Here's how the part is built. I have some questions about the finished solid (model axes, mm). A direction names the side the tool comes from. Coordinates: 2 decimals unless noted, no trailing zeros. Write each loop counter-clockwise with the first axis right and the second up, starting at its lowest first coordinate (ties: lowest second). Pieces come first, ordered by that corner, then holes.
Item 1: I want a section at A-A (y = 1.5). Please give me the cut outline in (x, z), and give its area (3 significant figures).
Item 2: For faces 4 (the face through (-28.503, 11.843, 0.986)), 5 (the face through (2, 14, 0)), which set-ups out of +Z, -Z, +X, -X, +Y, -Y let a thin tool reach every point of the face, with its end or its side?
Item 3: I want a section at B-B (z = 0.8). Please give me the cut outline in (x, y) (3 decimals).
Item 4: I'm going to push flat-ended pins straight in: P1, Ø1, axis at x = -28.5, z = 0.5, coming from the +Y side; P2, Ø1, axis at x = -10, z = 0.5, coming from the -Y side; P3, Ø1, axis at x = -34.5, z = 1.5, coming from the +Y side. Where does each tip first touch, or does it pass through?
Item 5: If we mould it in two halves opening along X, with no side actions, what happens to faces 1 (the face through (2, 11.896, 1)), 2 (the face through (63.977, 4, 1)), 3 (the face through (2, 14, 2))? For each: pulls with the +X half, pulls with the -X half, needs draft (parallel to the pull), parting line crosses it, or undercut.
Item 6: I want a section at C-C (y = 7). Please give me the cut outline in (x, z).
Item 7: I want a section at D-D (x = -3). Please give me the cut outline in (y, z), and give its area (3 significant figures).
Item 8: Please list where these lines run through material, in increasing order: line 1 (X direction, y = 3.25, z = 1.45); line 2 (Y direction, x = 13, z = 0.8); line 3 (Y direction, x = 34.5, z = 0.9).
from build123d import *

# Parameters (mm, degrees)
SALIENTE_EXTRUIR1_DEPTH = 2


with BuildPart() as part:
    # Croquis1 → Saliente-Extruir1 (new body)
    with BuildSketch(Plane.XY):
        with BuildLine():
            Line((-27.468702439, 15.986263571), (30.422317404, 15.986263571))
            ThreePointArc((30.422317404, 15.986263571), (31.470993229, 15.931125511), (32.508104664, 15.766319374))
            Line((32.508104664, 15.766319374), (63.185386208, 9.223791978))
            ThreePointArc((63.185386208, 9.223791978), (63.754167993, 8.874841751), (63.976807482, 8.245786398))
            Line((63.976807482, 8.245786398), (63.976807482, 0.055005987))
            ThreePointArc((63.976807482, 0.055005987), (63.683914264, -0.652100794), (62.976807482, -0.944994013))
            Line((62.976807482, -0.944994013), (62.176807482, -0.944994013))
            ThreePointArc((62.176807482, -0.944994013), (61.469700701, -0.652100794), (61.176807482, 0.055005987))
            Line((61.176807482, 0.055005987), (61.176807482, 4.752984684))
            ThreePointArc((61.176807482, 4.752984684), (60.954167993, 5.382040037), (60.385386208, 5.730990264))
            Line((60.385386208, 5.730990264), (32.508104664, 11.67636316))
            ThreePointArc((32.508104664, 11.67636316), (31.470993229, 11.841169298), (30.422317404, 11.896307357))
            Line((30.422317404, 11.896307357), (-27.468702439, 11.896307357))
            ThreePointArc((-27.468702439, 11.896307357), (-28.517378264, 11.841169298), (-29.554489699, 11.67636316))
            Line((-29.554489699, 11.67636316), (-57.431771244, 5.730990264))
            ThreePointArc((-57.431771244, 5.730990264), (-58.000553028, 5.382040037), (-58.223192518, 4.752984684))
            Line((-58.223192518, 4.752984684), (-58.223192518, 0.055005987))
            ThreePointArc((-58.223192518, 0.055005987), (-58.516085736, -0.652100794), (-59.223192518, -0.944994013))
            Line((-59.223192518, -0.944994013), (-60.023192518, -0.944994013))
            ThreePointArc((-60.023192518, -0.944994013), (-60.730299299, -0.652100794), (-61.023192518, 0.055005987))
            Line((-61.023192518, 0.055005987), (-61.023192518, 8.245786398))
            ThreePointArc((-61.023192518, 8.245786398), (-60.800553028, 8.874841751), (-60.231771244, 9.223791978))
            Line((-60.231771244, 9.223791978), (-29.554489699, 15.766319374))
            ThreePointArc((-29.554489699, 15.766319374), (-28.517378264, 15.931125511), (-27.468702439, 15.986263571))
        make_face()
    extrude(amount=SALIENTE_EXTRUIR1_DEPTH)


solid = part.part
Answer:
1. outline: (-61.02, 0) - (-58.22, 0) - (-58.22, 2) - (-61.02, 2) - close; (61.18, 0) - (63.98, 0) - (63.98, 2) - (61.18, 2) - close
1. area: 11.2 mm2
2. face 4: +Z, -Z, -Y
2. face 5: -Z, +X, -X, +Y, -Y
3. outline: (-61.023, 0.055) arc R1 ccw to (-60.023, -0.945) - (-59.223, -0.945) arc R1 ccw to (-58.223, 0.055) - (-58.223, 4.753) arc R1 cw to (-57.432, 5.731) - (-29.554, 11.676) arc R10 cw to (-27.469, 11.896) - (30.422, 11.896) arc R10 cw to (32.508, 11.676) - (60.385, 5.731) arc R1 cw to (61.177, 4.753) - (61.177, 0.055) arc R1 ccw to (62.177, -0.945) - (62.977, -0.945) arc R1 ccw to (63.977, 0.055) - (63.977, 8.246) arc R1 ccw to (63.185, 9.224) - (32.508, 15.766) arc R10 ccw to (30.422, 15.986) - (-27.469, 15.986) arc R10 ccw to (-29.554, 15.766) - (-60.232, 9.224) arc R1 ccw to (-61.023, 8.246) - close
4. P1: stops at y = 15.97
4. P2: stops at y = 11.9
4. P3: stops at y = 14.82
5. face 1: undercut
5. face 2: pulls with the +X half
5. face 3: needs draft
6. outline: (-61.02, 0) - (-51.48, 0) - (-51.48, 2) - (-61.02, 2) - close; (54.44, 0) - (63.98, 0) - (63.98, 2) - (54.44, 2) - close
7. outline: (11.9, 0) - (15.99, 0) - (15.99, 2) - (11.9, 2) - close
7. area: 8.18 mm2
8. line 1: x = -61.02 to -58.22, 61.18 to 63.98
8. line 2: y = 11.9 to 15.99
8. line 3: y = 11.25 to 15.34
